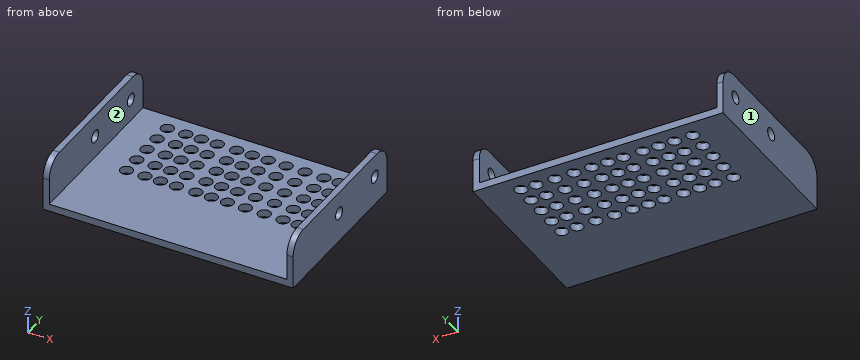
from build123d import *

# Parameters (mm, degrees)
F0_W      = 68
F0_H      = 29.5
F1_DEPTH  = 2
F2_W      = 1.9
F2_H      = 29.5
F3_DEPTH  = 12
F5_D      = 3.4
F7_D      = 3.4
F8_DEPTH  = 16.5
F9_DEPTH  = 0.2
F10_DEPTH = 0.2
F11_R     = 5


with BuildPart() as f1:
    # F0 (on Top) → F1 (new body)
    with BuildSketch(Plane.XY):
        Rectangle(F0_W, F0_H)
    extrude(amount=F1_DEPTH)

    # F2 (on face) → F3 (join)
    with BuildSketch(Plane.XY.offset(2)):
        with Locations((-33.05, 0)):
            Rectangle(F2_W, F2_H)
        with Locations((33.05, 0)):
            Rectangle(F2_W, F2_H)
    extrude(amount=F3_DEPTH)

    # F5 (through all)
    with Locations(Plane.YZ.offset(34)):
        with Locations((-8.75, 8), (8.75, 8)):
            Hole(F5_D / 2)

    # F7 (through all)
    with Locations(Plane(origin=(0, 0, 0), x_dir=(1, 0, 0), z_dir=(0, 0, -1))):
        with Locations((-23.0769233018, -10), (-18.076922571, -10), (-13.8461533964, -10), (-9.4871796933, -10), (-4.2307691746, -10), (0, -10), (4.3589744339, -10), (9.2307691746, -10), (14.3589744339, -10), (19.4871789625, -10), (23.5897428777, -10), (23.5897428777, -5), (19.4871789625, -5), (14.3589744339, -5), (9.2307691746, -5), (4.3589744339, -5), (0, -5), (-4.2307691746, -5), (-9.4871796933, -5), (-13.8461533964, -5), (-18.076922571, -5), (-23.0769233018, -5), (-23.0769233018, 0), (-18.076922571, 0), (-13.8461533964, 0), (-9.4871796933, 0), (-4.2307691746, 0), (0, 0), (14.3589744339, 0), (4.3589744339, 0), (9.2307691746, 0), (19.4871789625, 0), (23.5897428777, 0), (23.5897428777, 5), (19.4871789625, 5), (14.3589744339, 5), (9.2307691746, 5), (4.3589744339, 5), (0, 5), (-4.2307691746, 5), (-9.4871796933, 5), (-13.8461533964, 5), (-18.076922571, 5), (-23.0769233018, 5), (-23.0769233018, 10), (-18.076922571, 10), (-13.8461533964, 10), (-9.4871796933, 10), (-4.2307691746, 10), (0, 10), (4.3589744339, 10), (9.2307691746, 10), (14.3589744339, 10), (19.4871789625, 10), (23.5897428777, 10)):
            Hole(F7_D / 2)

    # F8 (add): a face of the model
    f8_faces = [f1.faces().sort_by_distance(p)[0] for p in [
        (-33.3057378017, -14.75, 7),
    ]]
    extrude(f8_faces, amount=F8_DEPTH)

    # F9 (cut): a face of the model
    f9_faces = [f1.faces().sort_by_distance(p)[0] for p in [
        (-32.1, -8.25, 2.475394573),
    ]]
    extrude(f9_faces, amount=-F9_DEPTH, mode=Mode.SUBTRACT)

    # F10 (cut): a face of the model
    f10_faces = [f1.faces().sort_by_distance(p)[0] for p in [
        (32.1, 14.274605427, 8),
    ]]
    extrude(f10_faces, amount=-F10_DEPTH, mode=Mode.SUBTRACT)

    # F11
    f11_edges = [f1.edges().sort_by_distance(p)[0] for p in [
        (-33.15, -31.25, 14),
        (33.15, -31.25, 14),
        (-33.15, 14.75, 14),
        (33.15, 14.75, 14),
    ]]
    fillet(f11_edges, radius=F11_R)


solid = f1.part
Check sheet for the modelled part. Datum: model origin and axes. Units: mm. Face numbers are marked on the shaded views. A direction names the side the tool comes from. Coordinates: 2 decimals unless noted, no trailing zeros. Loops run counter-clockwise (first coordinate to the right, second up) from the corner with the lowest first, then second, coordinate; pieces in that order, holes last. Notation, with made-up numbers: (-8, -30.5) -> (16, -30.5) arc R31 cw to (16, 5.5) -> close; hole circle Ø6 at (47.25, 6). An arc over 180 degrees is marked (long way). Answer in a Markdown table with one row per item.
1. Sectioned sample at B-B, the plane z = 3. Record the boundary of the cut face in (x, y), then the cut area to 3 significant figures.
Check values:
| item | result |
|---|---|
| outline | (-34, -31.25) -> (-32.3, -31.25) -> (-32.3, 14.75) -> (-34, 14.75) -> close; (32.3, -31.25) -> (34, -31.25) -> (34, 14.75) -> (32.3, 14.75) -> close |
| area | 156 mm2 |
2. Sectioned sample at D-D, the plane z = 12.5. Record the boundary of the cut face in (x, y), then the cut area to 3 significant figures.
Check values:
| item | result |
|---|---|
| outline | (-34, -29.82) -> (-32.3, -29.82) -> (-32.3, 13.32) -> (-34, 13.32) -> close; (32.3, -29.82) -> (34, -29.82) -> (34, 13.32) -> (32.3, 13.32) -> close |
| area | 147 mm2 |
3. Sectioned sample at A-A, the plane x = 0. Record the boundary of the cut face in (y, z), then the cut area to 3 significant figures.
Check values:
| item | result |
|---|---|
| outline | (-31.25, 0) -> (-11.7, 0) -> (-11.7, 2) -> (-31.25, 2) -> close; (-8.3, 0) -> (-6.7, 0) -> (-6.7, 2) -> (-8.3, 2) -> close; (-3.3, 0) -> (-1.7, 0) -> (-1.7, 2) -> (-3.3, 2) -> close; (1.7, 0) -> (3.3, 0) -> (3.3, 2) -> (1.7, 2) -> close; (6.7, 0) -> (8.3, 0) -> (8.3, 2) -> (6.7, 2) -> close; (11.7, 0) -> (14.75, 0) -> (14.75, 2) -> (11.7, 2) -> close |
| area | 58.0 mm2 |
4. Material ranges on line 1 along X through (y, z) = (-20.5, 10.5); line 2 along Y through (x, z) = (24, 1); line 3 along Z through (x, y) = (-18.5, -23.5), recorded low to high. Write a range as [from, to].
Check values:
| item | result |
|---|---|
| line 1 | x = [-34, -32.3], [32.3, 34] |
| line 2 | y = [-31.25, -11.65], [-8.35, -6.65], [-3.35, -1.65], [1.65, 3.35], [6.65, 8.35], [11.65, 14.75] |
| line 3 | z = [0, 2] |
5. Sectioned sample at C-C, the plane y = -23. Record the boundary of the cut face in (x, z).
Check values:
| item | result |
|---|---|
| outline | (-34, 0) -> (34, 0) -> (34, 14) -> (32.3, 14) -> (32.3, 2) -> (-32.3, 2) -> (-32.3, 14) -> (-34, 14) -> close |
6. Go/stop test with a flat-tipped pin: pin 1 (4 mm diameter, centred on x = -18.08, y = 0, fed in from +Z). Record where the tip stops, or that it passes through.
Check values:
| item | result |
|---|---|
| pin 1 | stops at z = 2 |
7. Access from +Z, -Z, +X, -X, +Y, -Y to the whole of each face (thin tool, end or side, straight path). Record for the marked faces 1 and 2.
Check values:
| item | result |
|---|---|
| face 1 | +Z, -Z, -X, +Y, -Y |
| face 2 | +Z, +Y, -Y |
